from build123d import *

# Parameters (mm, degrees)
SKETCH1_W           = 20
SKETCH1_H           = 200
BOSS_EXTRUDE1_DEPTH = 3
SKETCH2_W           = 3
SKETCH2_H           = 200
BOSS_EXTRUDE2_DEPTH = 170
CUT_EXTRUDE1_REACH  = 202.072
SKETCH3_R           = 2
LPATTERN1_COUNT     = 4
LPATTERN1_PITCH     = 60
CUT_EXTRUDE2_REACH  = 200.242
SKETCH4_R           = 2
LPATTERN2_COUNT     = 4
LPATTERN2_PITCH     = 60
SKETCH5_W           = 3
SKETCH5_H           = 10
BOSS_EXTRUDE3_DEPTH = 10
CUT_EXTRUDE3_REACH  = 264.679
SKETCH6_R           = 1.5


with BuildPart() as part:
    # Sketch1 → Boss-Extrude1 (new body)
    with BuildSketch(Plane(origin=(0, 0, 0), x_dir=(1, 0, 0), z_dir=(0, 1, 0))):
        Rectangle(SKETCH1_W, SKETCH1_H)
    extrude(amount=BOSS_EXTRUDE1_DEPTH)

    # Sketch2 → Boss-Extrude2 (add)
    with BuildSketch(Plane.XZ):
        with Locations((8.5, 0)):
            Rectangle(SKETCH2_W, SKETCH2_H)
    extrude(amount=BOSS_EXTRUDE2_DEPTH)

    # Sketch3 → Cut-Extrude1 (cut, up to next)
    with BuildSketch(Plane(origin=(0, 3, 0), x_dir=(1, 0, 0), z_dir=(0, 1, 0)), mode=Mode.PRIVATE) as cut_extrude1_sk1:
        with Locations(Location((0, -90, 0), (0, 0, 270))):
            Circle(SKETCH3_R)
    cut_extrude1_tool1 = extrude(cut_extrude1_sk1.sketch, amount=-CUT_EXTRUDE1_REACH, mode=Mode.PRIVATE) & part.part
    cut_extrude1 = cut_extrude1_tool1.solids().sort_by_distance((0, 3, 90))[0]
    add(cut_extrude1, mode=Mode.SUBTRACT)

    # LPattern1: Cut-Extrude1 ×4
    with Locations(*[(0, 0, -i * LPATTERN1_PITCH) for i in range(1, LPATTERN1_COUNT)]):
        add(cut_extrude1, mode=Mode.SUBTRACT)

    # Sketch4 → Cut-Extrude2 (cut, up to next)
    with BuildSketch(Plane(origin=(10, 0, 0), x_dir=(0, 0, -1), z_dir=(1, 0, 0)), mode=Mode.PRIVATE) as cut_extrude2_sk1:
        with Locations((90, -160)):
            Circle(SKETCH4_R)
    cut_extrude2_tool1 = extrude(cut_extrude2_sk1.sketch, amount=-CUT_EXTRUDE2_REACH, mode=Mode.PRIVATE) & part.part
    cut_extrude2 = cut_extrude2_tool1.solids().sort_by_distance((10, -160, -90))[0]
    add(cut_extrude2, mode=Mode.SUBTRACT)

    # LPattern2: Cut-Extrude2 ×4
    with Locations(*[(0, 0, i * LPATTERN2_PITCH) for i in range(1, LPATTERN2_COUNT)]):
        add(cut_extrude2, mode=Mode.SUBTRACT)

    # Sketch5 → Boss-Extrude3 (add)
    with BuildSketch(Plane.ZY.offset(-7)):
        with Locations((-98.5, -85)):
            Rectangle(SKETCH5_W, SKETCH5_H)
    boss_extrude3 = extrude(amount=BOSS_EXTRUDE3_DEPTH)

    # Sketch6 → Cut-Extrude3 (cut, up to next)
    with BuildSketch(Plane(origin=(0, 0, -100), x_dir=(-1, 0, 0), z_dir=(0, 0, -1)), mode=Mode.PRIVATE) as cut_extrude3_sk1:
        with Locations((-2, -85)):
            Circle(SKETCH6_R)
    cut_extrude3_tool1 = extrude(cut_extrude3_sk1.sketch, amount=-CUT_EXTRUDE3_REACH, mode=Mode.PRIVATE) & part.part
    cut_extrude3 = cut_extrude3_tool1.solids().sort_by_distance((2, -85, -100))[0]
    add(cut_extrude3, mode=Mode.SUBTRACT)

    # Mirror1: Boss-Extrude3, Cut-Extrude3 across plane
    add(boss_extrude3.mirror(Plane.XY))
    add(cut_extrude3.mirror(Plane.XY), mode=Mode.SUBTRACT)


solid = part.part
Can you work these out from the model? Positions are in its coordinate system, mm. A direction names the side the tool comes from. Give positions to 0.01 mm unless a question says otherwise; leave off trailing zeros. Order: outer loops, then holes, each group sorted by start corner. A loop starts at its lowest first (then second) coordinate and runs counter-clockwise, first axis right, second up. Notation, with made-up numbers: M -11,-35.75 L 25,-35.75 A20 ccw 25,-27.75 Z; hole C 70,82.25 d9. An arc over 180 degrees is marked long. Use a Markdown table: item, result. Add a question column.
Item 1: For faces 1 (the flat face through (3.2, -86.2, 97)), 2 (the cylindrical face through (8.521, -161.774, -90.923)), which set-ups out of +Z, -Z, +X, -X, +Y, -Y let a thin tool reach every point of the face, with its end or its side?
Item 2: If I drill on L1, parallel to X at y = 1, z = -30; L2, parallel to Y at x = 9.1, z = -30; L3, parallel to Z at x = 5.25, y = -81.5, over which ranges is the centre line in solid material (lowest first)? Write a range as [from, to].
Item 3: Will these pins go through, and if not, where does the flat tip stop? pin 1 (4 mm diameter, centred on x = -8, z = 46, fed in from -Y); pin 2 (4.5 mm diameter, centred on y = -160, z = 30, fed in from -X); pin 3 (6.5 mm diameter, centred on x = 0, z = -30, fed in from +Y); pin 4 (0.9 mm diameter, centred on y = -85, z = -98, fed in from -X).
Item 4: Suppose I cut it at A-A (z = 70). List the corners of the cut face in (x, y) for me, then the cut area to 3 significant figures.
Item 5: We'd pull the mould along X, two halves only. Please class faces 3 (the flat face through (10, -82, -1)), 4 (the cylindrical face through (0.601, 1.521, 91.908)), 5 (the cylindrical face through (0.601, 1.521, -88.092)), 6 (the flat face through (3.2, -86.2, -97)): +X half, -X half, draft (parallel to the pull), parting line (faces both ways), or undercut.
Item 6: Suppose I cut it at C-C (x = -7). List the corners of the cut face in (y, z) for me.
Item 7: Suppose I cut it at B-B (y = -143.5). List the corners of the cut face in (x, z) for me, then the cut area to 3 significant figures.
Answer sheet:
| question | item | result |
|---|---|---|
| 1 | face 1 | -X, -Y |
| 1 | face 2 | +X, -X |
| 2 | L1 | x = [-10, -2], [2, 10] |
| 2 | L2 | y = [-170, -162], [-158, 3] |
| 2 | L3 | z = [-100, -97], [97, 100] |
| 3 | pin 1 | stops at y = 0 |
| 3 | pin 2 | stops at x = 7 |
| 3 | pin 3 | stops at y = 3 |
| 3 | pin 4 | stops at x = -3 |
| 4 | outline | M -10,0 L 7,0 L 7,-170 L 10,-170 L 10,3 L -10,3 Z |
| 4 | area | 570 mm² |
| 5 | face 3 | +X half |
| 5 | face 4 | undercut |
| 5 | face 5 | undercut |
| 5 | face 6 | draft |
| 6 | outline | M 0,-100 L 3,-100 L 3,100 L 0,100 Z |
| 7 | outline | M 7,-100 L 10,-100 L 10,100 L 7,100 Z |
| 7 | area | 600 mm² |
